from build123d import *

# Parameters (mm, degrees)
F0_R     = 66.2228003741
F0_R_2   = 10
F1_DEPTH = 25
F0_R_3   = 97.356020809
F0_R_4   = 74.349079459
F2_DEPTH = 32
F4_SIZE  = 5
F5_SIZE  = 5


# Not quite as in the source:
# - a fillet or chamfer that OpenCascade refuses, or shapes differently, is made with other operations: its cross-section is extruded or revolved along the edge and cut away or added


with BuildPart() as f1:
    # F0 (on Right) → F1 (new body)
    with BuildSketch(Plane.YZ):
        Circle(F0_R)
        Circle(F0_R_2, mode=Mode.SUBTRACT)
    extrude(amount=F1_DEPTH)

    # F0 (on Right) → F2 (join)
    with BuildSketch(Plane.YZ):
        Circle(F0_R_3)
        Circle(F0_R_4, mode=Mode.SUBTRACT)
        Circle(F0_R_4)
        Circle(F0_R, mode=Mode.SUBTRACT)
    extrude(amount=F2_DEPTH)

    # F3: chamfer of 10 on 1 edges, made by hand


with BuildPart() as f3_tool2:
    # F3_s3 → F3_t4 (revolve)
    with BuildSketch(Plane.XY):
        Polygon((22, 66.2228003741), (32, 76.2228003741), (32, 66.2228003741), align=None)
    revolve(axis=Axis((32, 0, 0), (1, 0, 0)))

    split(bisect_by=Plane.YZ.offset(25), keep=Keep.TOP)


with BuildPart() as f1_1:
    add(f1.part)

    # F3_t1: cut F3_tool2
    add(f3_tool2.part, mode=Mode.SUBTRACT)

    # F4
    f4_edges = [f1_1.edges().sort_by_distance(p)[0] for p in [
        (32, -97.356021, 0),
    ]]
    chamfer(f4_edges, length=F4_SIZE)

    # F5
    f5_edges = [f1_1.edges().sort_by_distance(p)[0] for p in [
        (0, -97.356021, 0),
    ]]
    chamfer(f5_edges, length=F5_SIZE)


solid = f1_1.part
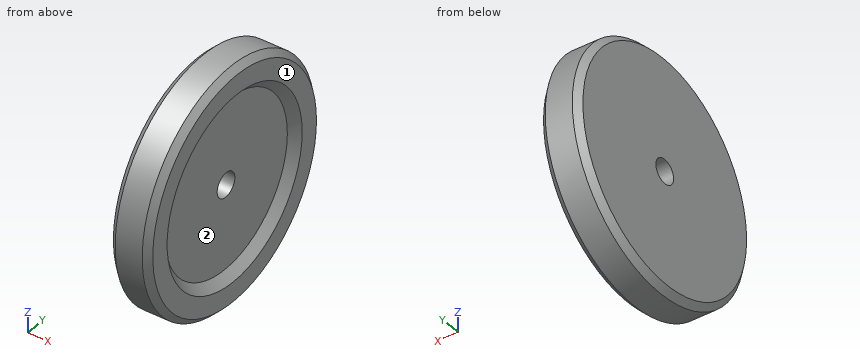
Verification items for the finished model (mm, model axes). Face numbers are marked on the shaded views. A direction names the side the tool comes from. Coordinates: 2 decimals unless noted, no trailing zeros. Order: outer loops, then holes, each group sorted by start corner. A loop starts at its lowest first (then second) coordinate and runs counter-clockwise, first axis right, second up. Notation, with made-up numbers: M 10,88.25 L 17,88.25 A25 ccw 17,114.25 Z; hole C 68.5,33 d7. An arc over 180 degrees is marked long. Return JSON: item names as keys, results as strings.
1) Gauge pin test, flat ends, axial feed: pin 1 (10 mm diameter, centred on x = 23.5, z = -13, fed in from +Y); pin 2 (1.5 mm diameter, centred on x = 28.5, z = 68, fed in from +Y); pin 3 (6 mm diameter, centred on x = 28, y = -41, fed in from +Z). Record the tip position at first contact, or that the pin passes through.
Answer list:
{"pin 1": "y = 97.03", "pin 2": "y = 68.85", "pin 3": "z = 89.56"}
2) Cross-section at C-C, the plane x = 9.5. Record the boundary of the cut face in (y, z).
Answer list:
{"outline": "C 0,0 d194.71; hole C 0,0 d20"}
3) Access from +Z, -Z, +X, -X, +Y, -Y to the whole of each face (thin tool, end or side, straight path). Record for the marked faces 1 and 2.
Answer list:
{"face 1": "+Z, -Z, +X, +Y, -Y", "face 2": "+X"}
4) Thickness scan on L1, parallel to Z at x = 19, y = 0; L2, parallel to X at y = 14, z = -34.5; L3, parallel to Z at x = 28.5, y = -12. Record the ranges inside material, lowest first. Write a range as [from, to].
Answer list:
{"L1": "[-97.36, -10], [10, 97.36]", "L2": "[0, 25]", "L3": "[-95.1, -71.73], [71.73, 95.1]"}
5) Cross-section at A-A, the plane y = 0. Record the boundary of the cut face in (x, z).
Answer list:
{"outline": "M 0,-92.36 L 5,-97.36 L 27,-97.36 L 32,-92.36 L 32,-76.22 L 25,-69.22 L 25,-10 L 0,-10 Z; M 0,10 L 25,10 L 25,69.22 L 32,76.22 L 32,92.36 L 27,97.36 L 5,97.36 L 0,92.36 Z"}
